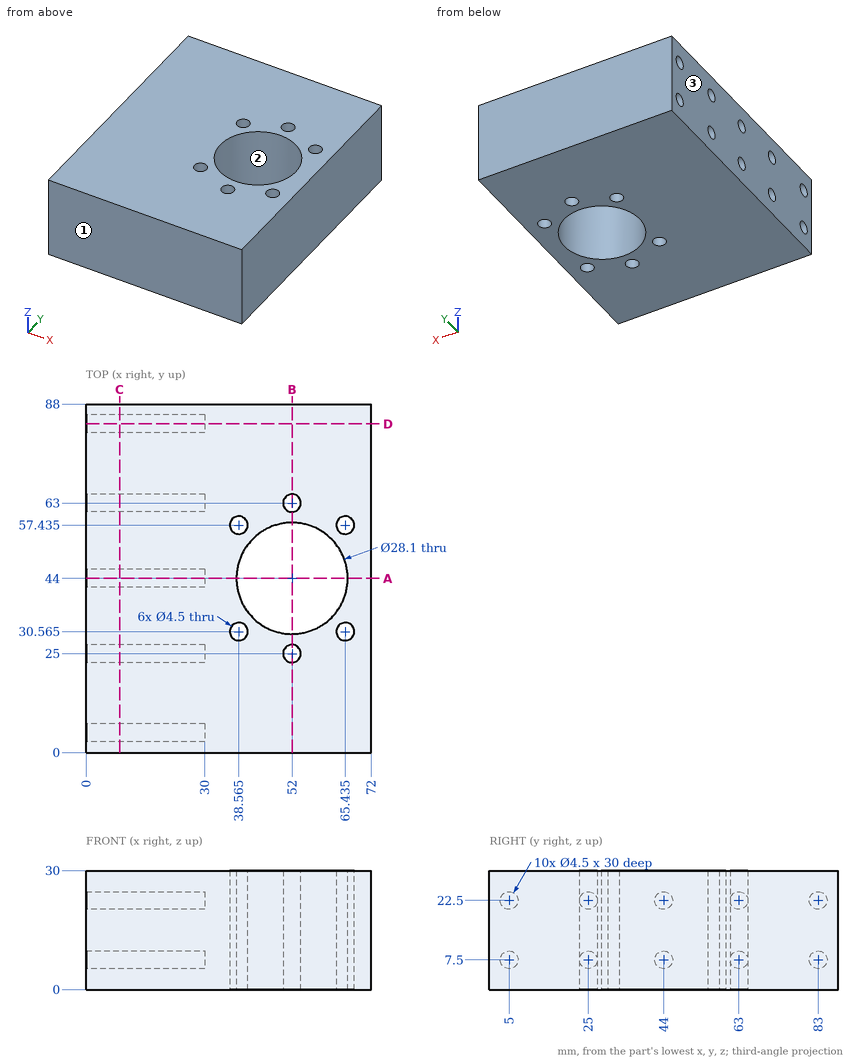
Design review of the part shown in the three views and the two pictorial views. Dimensions are in mm from the part's minimum x, y and z. Coordinates: 2 decimals unless noted, no trailing zeros. Write each loop counter-clockwise with the first axis right and the second up, starting at its lowest first coordinate (ties: lowest second). Pieces come first, ordered by that corner, then holes.
1) We need section B-B on x = 52. State the section outline as (y, z) points, then the cut area to 3 significant figures.
2) The part is to be moulded in two halves that separate along X. For the marked faces 1, 2 and 3, say which applies: pulls with the +X half, pulls with the -X half, needs draft (parallel to the pull), parting line crosses it, or undercut.
3) To check wall thickness, follow probe 1 along Y at (x, z) = (9, 22.5); probe 2 along Z at (x, y) = (14, 83); probe 3 along Y at (x, z) = (52, 11.25). State the ranges of each line that lie inside material, in increasing order.
4) We need section A-A on y = 44. State the section outline as (x, z) points, then the cut area to 3 significant figures.
5) We need section D-D on y = 83. State the section outline as (x, z) points.
6) We need section C-C on x = 8.5. Count the separate pieces of the cut face and the enclosed holes in it, then the cut area to 3 significant figures.
7) Clearance check with a flat-ended pin moving along its axis: pin 1 Ø2 at (y, z) = (44.5, 7.5) entering from -X. State where the tip first meets the part, or that it passes through.
Answer list:
1. outline: (0, 0) - (22.75, 0) - (22.75, 30) - (0, 30) - close; (27.25, 0) - (29.95, 0) - (29.95, 30) - (27.25, 30) - close; (58.05, 0) - (60.75, 0) - (60.75, 30) - (58.05, 30) - close; (65.25, 0) - (88, 0) - (88, 30) - (65.25, 30) - close
1. area: 1,530 mm2
2. face 1: needs draft
2. face 2: undercut
2. face 3: pulls with the -X half
3. probe 1: y = 0 to 2.75, 7.25 to 22.75, 27.25 to 41.75, 46.25 to 60.75, 65.25 to 80.75, 85.25 to 88
3. probe 2: z = 0 to 5.25, 9.75 to 20.25, 24.75 to 30
3. probe 3: y = 0 to 22.75, 27.25 to 29.95, 58.05 to 60.75, 65.25 to 88
4. outline: (0, 0) - (37.95, 0) - (37.95, 30) - (0, 30) - (0, 24.75) - (30, 24.75) - (30, 20.25) - (0, 20.25) - (0, 9.75) - (30, 9.75) - (30, 5.25) - (0, 5.25) - close; (66.05, 0) - (72, 0) - (72, 30) - (66.05, 30) - close
4. area: 1,050 mm2
5. outline: (0, 0) - (72, 0) - (72, 30) - (0, 30) - (0, 24.75) - (30, 24.75) - (30, 20.25) - (0, 20.25) - (0, 9.75) - (30, 9.75) - (30, 5.25) - (0, 5.25) - close
6. separate pieces: 1
6. enclosed holes: 10
6. area: 2,480 mm2
7. pin 1: stops at x = 30
